Autodesk Fusion 360 part; units mm, degrees
sketch "top hopper side" plane through (0, 0, 0) normal (0, 1, 0) x (1, 0, 0)
  line L0 (-76.2, 0) -> (0, 0)
  line L1 (0, 0) -> (-19.05, -19.05)
  line L2 (-19.05, -19.05) -> (-57.15, -19.05)
  line L3 (-57.15, -19.05) -> (-76.2, 0)
  dimension "d12" = 76.2
  dimension "d13" = 38.1
  dimension "d14" = 45
extrude "Extrude3" add sketch "top hopper side" along normal blind 234.95
sketch "side cutout" plane through (0, 0, 0) normal (0, -1, 0) x (1, 0, 0)
  line L0 (-19.05, 19.05) -> (-57.15, 19.05)
  line L1 (-57.15, 19.05) -> (-76.2, 0)
  line L2 (-76.2, 0) -> (0, 0)
  line L3 (0, 0) -> (-19.05, 19.05)
  line L4 (-76.2, 0) -> (-57.15, 19.05)
  line L5 (-19.05, 19.05) -> (0, 0)
  line L6 (-76.2, 0) -> (0, 0)
  line L7 (-57.15, 19.05) -> (-19.05, 19.05)
  line L8 (-73.1339, 1.27) -> (-3.0661, 1.27)
  line L9 (-19.5761, 17.78) -> (-3.0661, 1.27)
  line L10 (-56.6239, 17.78) -> (-19.5761, 17.78)
  line L11 (-73.1339, 1.27) -> (-56.6239, 17.78)
  dimension "d17" = 1.27
extrude "Extrude4" cut sketch "side cutout" against normal blind 228.6 contours L8 L9 L10 L11
sketch "bottom cutout" plane through (0, 0, 0) normal (0, 0, -1) x (1, 0, 0)
  line L0 (0, 0) -> (-76.2, 0)
  line L1 (-76.2, 0) -> (-76.2, -234.95)
  line L2 (-76.2, -234.95) -> (0, -234.95)
  line L3 (0, -234.95) -> (0, 0)
  line L4 (-5.08, -5.08) -> (-70.7474, -5.08)
  line L5 (-70.7474, -5.08) -> (-70.7474, -228.6)
  line L6 (-5.08, -228.6) -> (-5.08, -5.08)
  line L7 (-5.08, -228.6) -> (-70.7474, -228.6)
  dimension "d20" = 223.52
  dimension "d21" = 65.6674
  dimension "d22" = 5.08
  dimension "d23" = 5.08
extrude "Extrude5" cut sketch "bottom cutout" against normal blind 2.54 contours L4 L5 L6 L7
sketch "top cutout" plane through (0, 0, 19.05) normal (0, 0, 1) x (-1, 0, 0)
  line L0 (57.15, 0) -> (19.05, 0)
  line L1 (19.05, 0) -> (19.05, -234.95)
  line L2 (19.05, -234.95) -> (57.15, -234.95)
  line L3 (57.15, -234.95) -> (57.15, 0)
  line L4 (53.34, -2.54) -> (22.86, -2.54)
  line L5 (22.86, -2.54) -> (22.86, -231.14)
  line L6 (22.86, -231.14) -> (53.34, -231.14)
  line L7 (53.34, -231.14) -> (53.34, -2.54)
  dimension "d26" = 228.6
  dimension "d27" = 30.48
  dimension "d28" = 3.81
  dimension "d29" = 2.54
extrude "Extrude6" cut sketch "top cutout" against normal blind 5.08 contours L4 L5 L6 L7

Autodesk Fusion 360 part; units mm, degrees
sketch "wheel" plane through (0, 0, 0) normal (0, 0, 1) x (1, 0, 0)
  circle A0 centre (0, 0) radius 19.05
  line L0 (-3.1964, 18.7799) -> (-3.1964, 22.86)
  line L1 (-3.1964, 22.86) -> (3.1964, 22.86)
  line L2 (3.1964, 22.86) -> (3.1964, 18.7799)
  line L3 (-13.6245, 13.3144) -> (-16.0227, 16.6153)
  line L4 (-16.0227, 16.6153) -> (-10.8508, 20.3729)
  line L5 (-10.8508, 20.3729) -> (-8.4526, 17.0721)
  line L6 (-18.8485, 2.7633) -> (-22.7289, 4.0241)
  line L7 (-22.7289, 4.0241) -> (-20.7534, 10.1041)
  line L8 (-20.7534, 10.1041) -> (-16.873, 8.8433)
  line L9 (-16.873, -8.8433) -> (-20.7534, -10.1041)
  line L10 (-20.7534, -10.1041) -> (-22.7289, -4.0241)
  line L11 (-22.7289, -4.0241) -> (-18.8485, -2.7633)
  line L12 (-8.4526, -17.0721) -> (-10.8508, -20.373)
  line L13 (-10.8508, -20.373) -> (-16.0227, -16.6153)
  line L14 (-16.0227, -16.6153) -> (-13.6245, -13.3145)
  line L15 (3.1964, -18.7799) -> (3.1964, -22.86)
  line L16 (3.1964, -22.86) -> (-3.1964, -22.86)
  line L17 (-3.1964, -22.86) -> (-3.1964, -18.7799)
  line L18 (13.6245, -13.3144) -> (16.0227, -16.6153)
  line L19 (16.0227, -16.6153) -> (10.8508, -20.3729)
  line L20 (10.8508, -20.3729) -> (8.4526, -17.0721)
  line L21 (18.8485, -2.7633) -> (22.7289, -4.0241)
  line L22 (22.7289, -4.0241) -> (20.7534, -10.1041)
  line L23 (20.7534, -10.1041) -> (16.873, -8.8433)
  line L24 (16.873, 8.8433) -> (20.7534, 10.1041)
  line L25 (20.7534, 10.1041) -> (22.7289, 4.0241)
  line L26 (22.7289, 4.0241) -> (18.8485, 2.7633)
  line L27 (8.4526, 17.0721) -> (10.8508, 20.373)
  line L28 (10.8508, 20.373) -> (16.0227, 16.6153)
  line L29 (16.0227, 16.6153) -> (13.6245, 13.3145)
  dimension "d1" = 38.1
  dimension "d2" = 6.3929
  dimension "d3" = 4.0801
  dimension "d5" = 360
extrude "Extrude1" add sketch "wheel" along normal blind 3.81
sketch "hole punch" plane through (0, 0, 3.81) normal (0, 0, 1) x (-1, 0, 0)
  arc A0 (-8.4526, -17.0721) -> (-3.1964, -18.7799) centre (0, 0) ccw
  line L0 (-3.1964, -18.7799) -> (-3.1964, -22.86)
  line L1 (-3.1964, -22.86) -> (3.1964, -22.86)
  line L2 (3.1964, -22.86) -> (3.1964, -18.7799)
  arc A1 (3.1964, -18.7799) -> (8.4526, -17.0721) centre (0, 0) ccw
  line L3 (8.4526, -17.0721) -> (10.8508, -20.3729)
  line L4 (10.8508, -20.3729) -> (16.0227, -16.6153)
  line L5 (16.0227, -16.6153) -> (13.6245, -13.3144)
  arc A2 (13.6245, -13.3144) -> (16.873, -8.8433) centre (0, 0) ccw
  line L6 (16.873, -8.8433) -> (20.7534, -10.1041)
  line L7 (20.7534, -10.1041) -> (22.7289, -4.0241)
  line L8 (22.7289, -4.0241) -> (18.8485, -2.7633)
  arc A3 (18.8485, -2.7633) -> (18.8485, 2.7633) centre (0, 0) ccw
  line L9 (18.8485, 2.7633) -> (22.7289, 4.0241)
  line L10 (22.7289, 4.0241) -> (20.7534, 10.1041)
  line L11 (20.7534, 10.1041) -> (16.873, 8.8433)
  arc A4 (16.873, 8.8433) -> (13.6245, 13.3145) centre (0, 0) ccw
  line L12 (13.6245, 13.3145) -> (16.0227, 16.6153)
  line L13 (16.0227, 16.6153) -> (10.8508, 20.373)
  line L14 (10.8508, 20.373) -> (8.4526, 17.0721)
  arc A5 (8.4526, 17.0721) -> (3.1964, 18.7799) centre (0, 0) ccw
  line L15 (3.1964, 18.7799) -> (3.1964, 22.86)
  line L16 (3.1964, 22.86) -> (-3.1964, 22.86)
  line L17 (-3.1964, 22.86) -> (-3.1964, 18.7799)
  arc A6 (-3.1964, 18.7799) -> (-8.4526, 17.0721) centre (0, 0) ccw
  line L18 (-8.4526, 17.0721) -> (-10.8508, 20.3729)
  line L19 (-10.8508, 20.3729) -> (-16.0227, 16.6153)
  line L20 (-16.0227, 16.6153) -> (-13.6245, 13.3144)
  arc A7 (-13.6245, 13.3144) -> (-16.873, 8.8433) centre (0, 0) ccw
  line L21 (-16.873, 8.8433) -> (-20.7534, 10.1041)
  line L22 (-20.7534, 10.1041) -> (-22.7289, 4.0241)
  line L23 (-22.7289, 4.0241) -> (-18.8485, 2.7633)
  arc A8 (-18.8485, 2.7633) -> (-18.8485, -2.7633) centre (0, 0) ccw
  line L24 (-18.8485, -2.7633) -> (-22.7289, -4.0241)
  line L25 (-22.7289, -4.0241) -> (-20.7534, -10.1041)
  line L26 (-20.7534, -10.1041) -> (-16.873, -8.8433)
  arc A9 (-16.873, -8.8433) -> (-13.6245, -13.3145) centre (0, 0) ccw
  line L27 (-13.6245, -13.3145) -> (-16.0227, -16.6153)
  line L28 (-16.0227, -16.6153) -> (-10.8508, -20.373)
  line L29 (-10.8508, -20.373) -> (-8.4526, -17.0721)
  circle A10 centre (0, 0) radius 19.05
  line L30 (0.0528, -19.0499) -> (0.0528, 19.0499)
  line L31 (19.05, 0) -> (-19.05, 0)
hole "Hole1" at (0, 0, 3.81) direction (0, 0, -1) diameter 6.2 depth 6.2 tip angle 118
The model under review builds one solid part; all positions refer to its coordinate system, in mm. A direction names the side the tool comes from. Round coordinates to 2 decimals unless told otherwise and drop trailing zeros. Loops run counter-clockwise (first coordinate to the right, second up) from the corner with the lowest first, then second, coordinate; pieces in that order, holes last. Notation, with made-up numbers: (67.5, 71.5) -> (77.5, 71.5) arc R24 ccw to (77.5, 96.5) -> close; hole circle Ø1 at (10.25, 71). An arc over 180 degrees is marked (long way). One line per question, with ' | ' between items. Start each with the question number.
Item 1: Add section A-A, the plane x = -45. Write out the cut boundary in (y, z).
Item 2: Add section C-C, the plane z = 8. Write out the cut boundary in (x, y).
Item 3: Add section B-B, the plane y = 29. Write out the cut boundary in (x, z), then the cut area to 3 significant figures.
Item 4: For pin 1 (1.9 mm diameter, centred on y = 20.5, z = 1.5, fed in from +X); pin 2 (1.5 mm diameter, centred on x = -34.5, z = 16.5, fed in from -Y); pin 3 (7 mm diameter, centred on x = 0, y = 0, fed in from +Z), all flat-tipped, find the tip position at first contact; note any pin that passes through.
Item 5: Machinability: for faces 5 (the face through (-38, 231.14, 17)), 6 (the face through (-54, 117, 19.05)), which of the approach directions +Z, -Z, +X, -X, +Y, -Y give a long, thin tool a straight path to every point of the face, cutting with its end or side? Answer none if there is none.
Item 6: Draft analysis for pull direction Y (two halves, no side actions). For faces 1 (the face through (-9, 116, 9)), 2 (the face through (2.75, -1.43, 1.88)), 3 (the face through (-53.34, 117.4, 18.6)), 4 (the face through (-39, 234.95, 7)), state which applies: +Y half, -Y half, draft (parallel to the pull), parting line (faces both ways), or undercut.
Item 7: Wall thickness on line 1 along Y through (x, z) = (-44.5, 1); line 2 along Y through (x, z) = (0, 2.55); line 3 along X through (y, z) = (147, 3.5): over which ranges is each line inside the solid? List them lowest first. Write a range as [from, to].
Return value:
1) outline: (0, 0) -> (5.08, 0) -> (5.08, 1.27) -> (0, 1.27) -> close; (0, 17.78) -> (2.54, 17.78) -> (2.54, 19.05) -> (0, 19.05) -> close; (228.6, 0) -> (234.95, 0) -> (234.95, 19.05) -> (231.14, 19.05) -> (231.14, 13.97) -> (228.6, 13.97) -> close
2) outline: (-68.2, 0) -> (-66.4, 0) -> (-66.4, 228.6) -> (-9.8, 228.6) -> (-9.8, 0) -> (-8, 0) -> (-8, 234.95) -> (-68.2, 234.95) -> close
3) outline: (-76.2, 0) -> (-70.75, 0) -> (-70.75, 1.27) -> (-73.13, 1.27) -> (-56.62, 17.78) -> (-53.34, 17.78) -> (-53.34, 19.05) -> (-57.15, 19.05) -> close; (-22.86, 17.78) -> (-19.58, 17.78) -> (-3.07, 1.27) -> (-5.08, 1.27) -> (-5.08, 0) -> (0, 0) -> (-19.05, 19.05) -> (-22.86, 19.05) -> close | area: 82.4 mm2
4) pin 1: stops at x = 11.98 | pin 2: stops at y = 231.14 | pin 3: stops at z = 3.81
5) face 5: +Z | face 6: +Z, +X, -X, +Y, -Y
6) face 1: draft | face 2: undercut | face 3: undercut | face 4: +Y half
7) line 1: y = [0, 5.08], [228.6, 234.95] | line 2: y = [-22.86, -3.1], [3.1, 22.86] | line 3: x = [-72.7, -70.9], [-5.3, -3.5]
